Can you work these out from the drawing? Everything is in mm from the part's minimum corner. A direction names the side the tool comes from. Give positions to 0.01 mm unless a question says otherwise; leave off trailing zeros. Loops run counter-clockwise (first coordinate to the right, second up) from the corner with the lowest first, then second, coordinate; pieces in that order, holes last. Notation, with made-up numbers: M 58.25,18.5 L 67.25,18.5 A10 ccw 67.25,28.5 Z; hole C -16.75,6.25 d11. An arc over 180 degrees is marked long. Use CSV: the item, a comma, the result in double quotes.
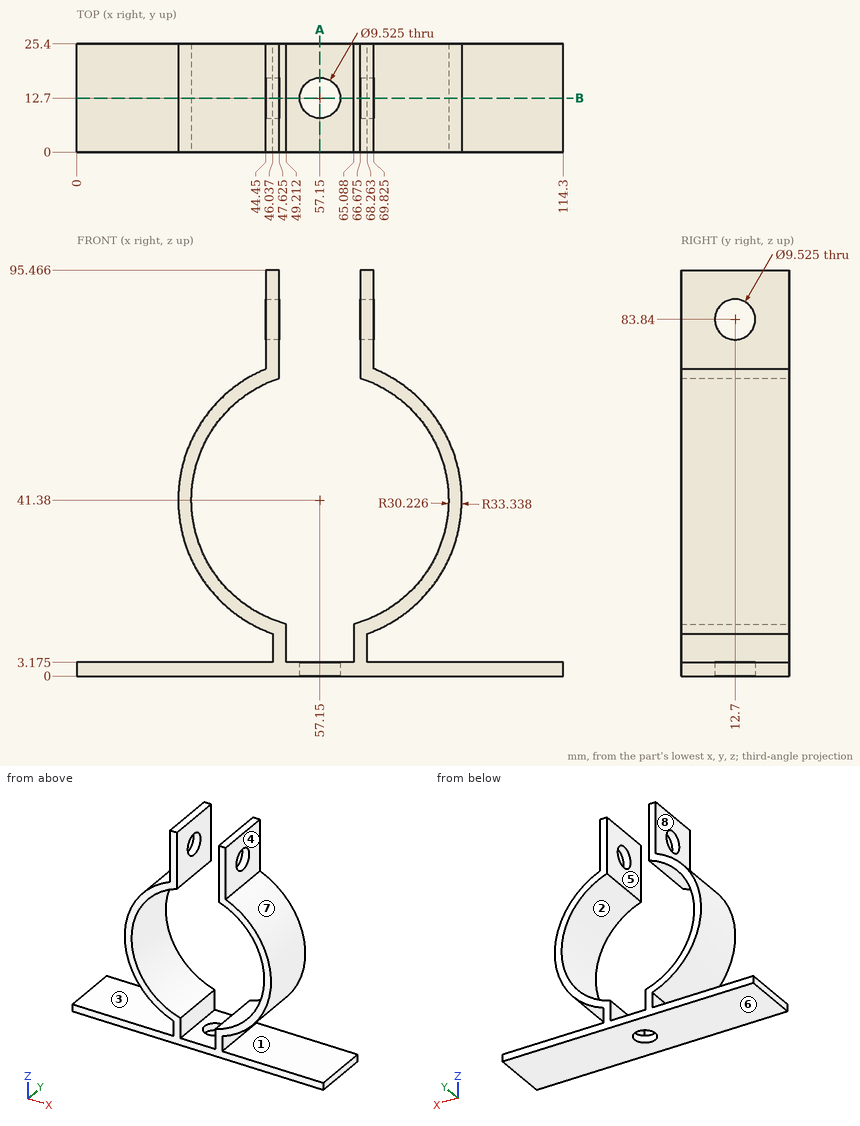
Q1. If we mould it in two halves opening along Z, with no side actions, what happens to the marked faces 6, 7 and 8? For each: released by +Z, released by -Z, zero draft, split by the parting line, or undercut.
Model answer:
face 6,"released by -Z"
face 7,"undercut"
face 8,"zero draft"
Q2. I want a section at B-B, the plane y = 12.7. State how many separate pieces and enclosed holes the cut face has.
Model answer:
separate pieces,"4"
enclosed holes,"0"
Q3. For the marked faces 1, 2, 3, 4 and 5, which set-ups out of +Z, -Z, +X, -X, +Y, -Y let a thin tool reach every point of the face, with its end or its side?
Model answer:
face 1,"+X, +Y, -Y"
face 2,"+Y, -Y"
face 3,"-X, +Y, -Y"
face 4,"+Z, +X, +Y, -Y"
face 5,"+Z, +Y, -Y"
Q4. I'm going to push flat-ended pins straight in: P1, Ø5, axis at y = 19.5, z = 71, coming from the -X side; P2, Ø6, axis at y = 18.5, z = 48, coming from the +X side; P3, Ø5, axis at x = 88, y = 8, coming from the +Z side; P4, Ø10, axis at x = 51, z = 63.5, coming from the +Y side. Where does each tip first touch, or does it pass through?
Model answer:
P1,"x = 37.76"
P2,"x = 90.29"
P3,"z = 58.92"
P4,"through"
Q5. I want a section at A-A, the plane x = 57.15. Please give me the cut outline in (y, z) (1 decimal), then the cut area to 3 significant figures.
Model answer:
outline,"M 0,0 L 7.9,0 L 7.9,3.2 L 0,3.2 Z; M 17.5,0 L 25.4,0 L 25.4,3.2 L 17.5,3.2 Z"
area,"50.4 mm2"
Q6. Please list where these lines run through material, in increasing order: L1, parallel to X at y = 12, z = 5.5; L2, parallel to Z at x = 83, y = 19.75 (1 decimal); L3, parallel to Z at x = 42, y = 12 (1 decimal). Write a range as from..to.
Model answer:
L1,"46.04..49.21, 65.09..68.26"
L2,"0..3.2, 20.3..25.7, 57..62.4"
L3,"0..3.2, 11.7..15.2, 67.5..71.1"
